Autodesk Inventor part; units mm, degrees
ref_plane "YZ Plane" through (0, 0, 0) normal (1, 0, 0) x (0, 1, 0)
ref_plane "XZ Plane" through (0, 0, 0) normal (0, 1, 0) x (-1, 0, 0)
ref_plane "XY Plane" through (0, 0, 0) normal (0, 0, 1) x (1, 0, 0)
sketch "スケッチ1" plane through (0, 0, 0) normal (0, 0, 1) x (1, 0, 0)
  line L0 (7.5, -7.5) -> (-7.5, -7.5)
  line L1 (-7.5, -7.5) -> (-7.5, 7.5)
  line L2 (-7.5, 7.5) -> (7.5, 7.5)
  line L3 (7.5, 7.5) -> (7.5, -7.5)
  line L4 (7.5, -7.5) -> (-7.5, 7.5) construction
  line L5 (-7.5, -7.5) -> (7.5, 7.5) construction
  line L6 (-7.5, 0) -> (7.5, 0) construction
  line L7 (6.5, 6.5) -> (-6.5, 6.5)
  line L8 (-6.5, 6.5) -> (-6.5, -6.5)
  line L9 (-6.5, -6.5) -> (6.5, -6.5)
  line L10 (6.5, -6.5) -> (6.5, 6.5)
  point P0 (0, 0)
  dimension "d0" = 15
  dimension "d1" = 15
  dimension "d2" = 1
extrude "押し出し1" add sketch "スケッチ1" along normal blind 32
sketch "スケッチ2" plane through (7.5, -7.5, 0) normal (1, 0, 0) x (0, 0, -1)
  line L0 (0, 15) -> (0, 0)
  line L1 (0, 15) -> (-32, 15)
  line L2 (-32, 0) -> (-32, 15)
  line L3 (0, 0) -> (-32, 0)
  line L4 (-32, 7.5) -> (0, 7.5) construction
  line L5 (-16, 7.5) -> (-16, 15) construction
  circle A0 centre (-29, 7.5) radius 3 construction
  circle A1 centre (-29, 7.5) radius 1.6
  circle A2 centre (-3, 7.5) radius 3 construction
  circle A3 centre (-3, 7.5) radius 1.6
  dimension "d5" = 6
  dimension "d6" = 3.2
extrude "押し出し2" cut sketch "スケッチ2" against normal through all contours A1 | A3
sketch "スケッチ3" plane through (-7.5, 7.5, 0) normal (0, 1, 0) x (1, 0, 0)
  line L0 (0, 0) -> (15, 0)
  line L1 (0, 0) -> (0, -32)
  line L2 (15, -32) -> (0, -32)
  line L3 (15, 0) -> (15, -32)
  line L4 (7.5, 0) -> (7.5, -32) construction
  line L5 (15, -16) -> (0, -16) construction
  circle A0 centre (7.5, -10) radius 1.6
  circle A1 centre (7.5, -22) radius 1.6
  dimension "d9" = 3.2
  dimension "d10" = 6
extrude "押し出し3" cut sketch "スケッチ3" against normal through all contours A0 | A1
properties part number "支え角柱(サーボ用)" material "アルミニウム 6061"
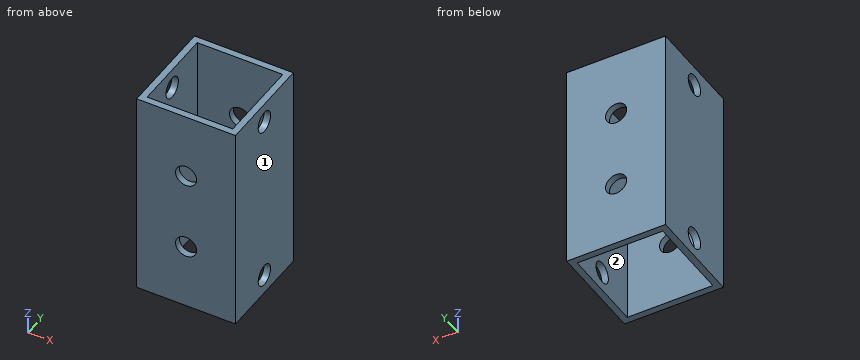
Could you check a few things on this model? Use its own coordinates, in mm. Face numbers are marked on the shaded views. A direction names the side the tool comes from. Round coordinates to 2 decimals unless told otherwise and drop trailing zeros. Write each loop counter-clockwise with the first axis right and the second up, starting at its lowest first coordinate (ties: lowest second). Pieces come first, ordered by that corner, then holes. Notation, with made-up numbers: (-9, 38.25) - (12, 38.25) arc R9 ccw to (12, 50.25) - close; hole circle Ø9 at (-24.75, -3). An arc over 180 degrees is marked (long way). Put each result on its own line as item: value. Start each with the question number.
(1) For the marked faces 1 and 2, which set-ups out of +Z, -Z, +X, -X, +Y, -Y let a thin tool reach every point of the face, with its end or its side?
(2) Will these pins go through, and if not, where does the flat tip stop? pin 1 (4 mm diameter, centred on x = 0, z = 22, fed in from -Y); pin 2 (1.9 mm diameter, centred on x = 0, z = 22, fed in from +Y).
(3) I want a section at D-D, the plane z = 5. Please give me the cut outline in (x, y).
(4) I want a section at A-A, the plane y = 3.25. Please give me the cut outline in (x, z), plus the area to 3 significant figures.
(5) I want a section at B-B, the plane z = 29. Please give me the cut outline in (x, y).
(6) I need wall thicknesses on probe 1 along Y at (x, z) = (1, 29); probe 2 along Y at (x, z) = (-7, 3). Which ranges of each line are inside material? Lowest first, please.
Here are the results:
1. face 1: +Z, -Z, +X, +Y, -Y
1. face 2: +Z, -Z
2. pin 1: stops at y = -7.5
2. pin 2: passes through
3. outline: (-7.5, -7.5) - (7.5, -7.5) - (7.5, 7.5) - (-7.5, 7.5) - close; hole (-6.5, -6.5) - (6.5, -6.5) - (6.5, 6.5) - (-6.5, 6.5) - close
4. outline: (-7.5, 0) - (-6.5, 0) - (-6.5, 32) - (-7.5, 32) - close; (6.5, 0) - (7.5, 0) - (7.5, 32) - (6.5, 32) - close
4. area: 64.0 mm^2
5. outline: (-7.5, -7.5) - (7.5, -7.5) - (7.5, -1.6) - (6.5, -1.6) - (6.5, -6.5) - (-6.5, -6.5) - (-6.5, -1.6) - (-7.5, -1.6) - close; (-7.5, 1.6) - (-6.5, 1.6) - (-6.5, 6.5) - (6.5, 6.5) - (6.5, 1.6) - (7.5, 1.6) - (7.5, 7.5) - (-7.5, 7.5) - close
6. probe 1: y = -7.5 to -6.5, 6.5 to 7.5
6. probe 2: y = -7.5 to -1.6, 1.6 to 7.5
